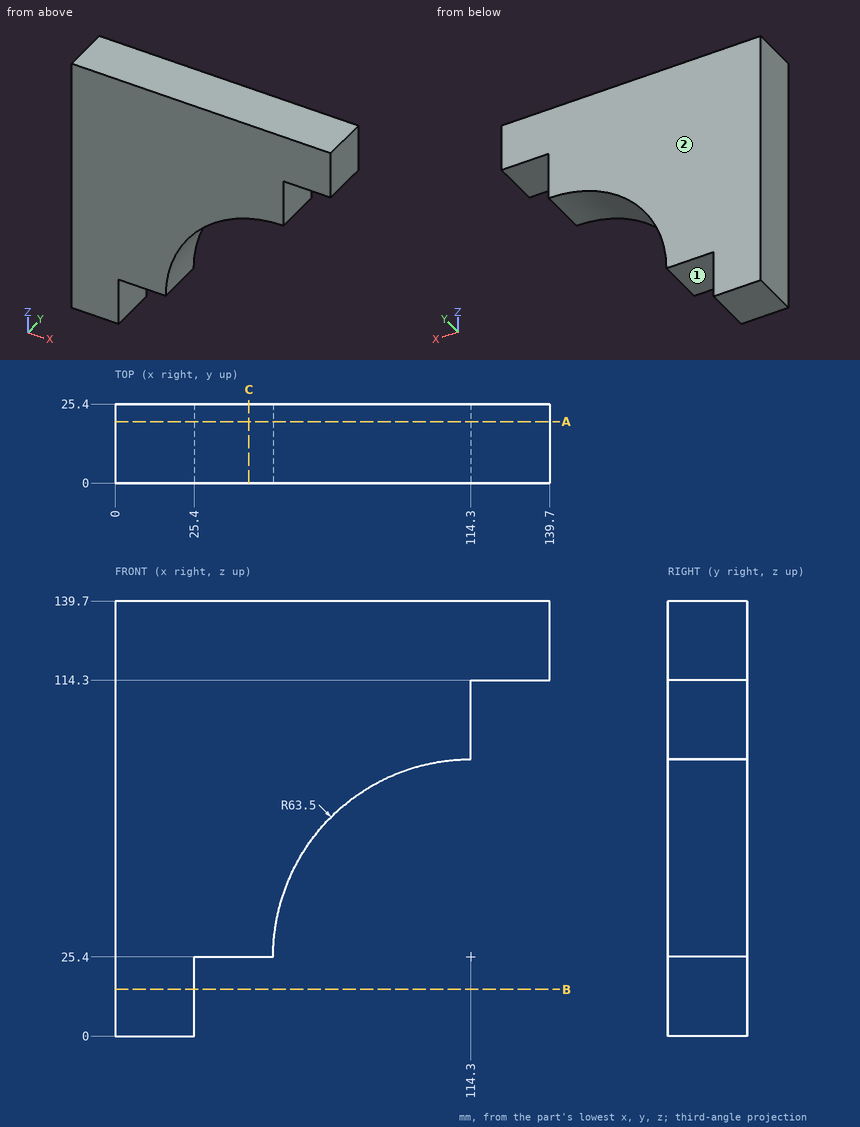
Can you work these out from the drawing? Everything is in mm from the part's minimum corner. A direction names the side the tool comes from. Coordinates: 2 decimals unless noted, no trailing zeros. Order: outer loops, then holes, each group sorted by start corner. A loop starts at its lowest first (then second) coordinate and runs counter-clockwise, first axis right, second up. Notation, with made-up numbers: M 12.5,0 L 20.5,0 A23 ccw 20.5,32 Z; hole C 20,14 d6. An arc over 180 degrees is marked long. Answer as CSV lines item,"result". Start each with the question number.
1. I want a section at A-A, the plane y = 19.75. Write out the boundary of the cut face in (x, z).
2. I need wall thicknesses on line 1 (X direction, y = 24.25, z = 103.5); line 2 (Z direction, x = 27, y = 15); line 3 (X direction, y = 5, z = 15.5). Which ranges of each line are inside material? Lowest first, please. Write a range as [from, to].
3. I want a section at C-C, the plane x = 43. Write out the boundary of the cut face in (y, z), and give its area (3 significant figures).
4. I want a section at B-B, the plane z = 15. Write out the boundary of the cut face in (x, y).
5. On a 3-axis mill with a long thin cutter (end or side, diameter ignored), from which of +Z, -Z, +X, -X, +Y, -Y can I reach the whole of each face in a straight line? I mean the marked faces 1 and 2. Say none if no direction works.
6. For pin 1 (12 mm diameter, centred on y = 15, z = 69.5, fed in from +X); pin 2 (1.5 mm diameter, centred on x = 106.5, y = 10.5, fed in from -Z); pin 3 (12.5 mm diameter, centred on x = 131, y = 19, fed in from -Z); pin 4 (2 mm diameter, centred on x = 29, z = 49, fed in from -Y), each with a flat end and sliding along its axis, tell me the tip position at first contact or that it passes through.
Recorded:
1,outline,"M 0,0 L 25.4,0 L 25.4,25.4 L 50.8,25.4 A63.5 cw 114.3,88.9 L 114.3,114.3 L 139.7,114.3 L 139.7,139.7 L 0,139.7 Z"
2,line 1,"x = [0, 114.3]"
2,line 2,"z = [25.4, 139.7]"
2,line 3,"x = [0, 25.4]"
3,outline,"M 0,25.4 L 25.4,25.4 L 25.4,139.7 L 0,139.7 Z"
3,area,"2,900 mm2"
4,outline,"M 0,0 L 25.4,0 L 25.4,25.4 L 0,25.4 Z"
5,face 1,"-Z, +X, +Y, -Y"
5,face 2,"+Z, -Z, +X, -X, +Y"
6,pin 1,"stops at x = 75.28"
6,pin 2,"stops at z = 88.32"
6,pin 3,"stops at z = 114.3"
6,pin 4,"stops at y = 0"
